Read the model definition and answer for the solid it produces. Units are mm, in the model's axes. A direction names the side the tool comes from. Coordinates: 2 decimals unless noted, no trailing zeros. Order: outer loops, then holes, each group sorted by start corner. A loop starts at its lowest first (then second) coordinate and runs counter-clockwise, first axis right, second up. Notation, with made-up numbers: M 18.5,-26 L 49.5,-26 A13 ccw 49.5,-15 Z; hole C 55.25,2.25 d5. An arc over 180 degrees is marked long. Put each result on its own line as item: value.
Autodesk Inventor part; units mm, degrees
ref_plane "Work Plane1" through (30, 0, 0) normal (0, -0.5, 0.866) x (1, 0, 0)
ref_plane "YZ Plane" through (0, 0, 0) normal (1, 0, 0) x (0, 1, 0)
ref_plane "XZ Plane" through (0, 0, 0) normal (0, 1, 0) x (-1, 0, 0)
sketch "Esquisse1" plane through (0, 0, 0) normal (0, 0, 1) x (1, 0, 0)
  line L0 (-1.1667, 0) -> (20, 0)
  line L1 (20, 0) -> (20, 2.5)
  line L2 (20, 2.5) -> (1.4815, 2.5)
  line L3 (1.4815, 2.5) -> (0.9908, 2.5)
  line L4 (0.9908, 2.5) -> (0, 2.5)
  line L5 (0, 2.5) -> (0, 4.25)
  line L6 (0, 4.25) -> (-5, 4.25)
  line L7 (-5, 4.25) -> (-5, 2.3094)
  line L8 (-5, 2.3094) -> (-2.5, 2.3094)
  line L9 (-2.5, 2.3094) -> (-1.1667, 0)
  line L10 (-10, 0) -> (25, 0)
  line L11 (0, -0.85) -> (0, 5.1)
  line L12 (1.4815, 2.5) -> (0, 2.5) construction
  dimension "d0" = 18.5185
  dimension "d1" = 0.4908
  dimension "d2" = 5
  dimension "d3" = 2.5
  dimension "d4" = 60
  dimension "d5" = 5
  dimension "d6" = 5
  dimension "d7" = 4.6188
  dimension "d8" = 8.5
  dimension "d19" = 20
revolve "Corps" add sketch "Esquisse1" angle 360 about axis through (-1.1667, 0, 0) along (1, 0, 0)
sketch "Esquisse2" plane through (-5, 0, 0) normal (-1, 0, 0) x (0, 0, 1)
  circle A0 centre (0, 0) radius 2.3094
  line L0 (0, -5.95) -> (0, 5.95)
  line L1 (-5.95, 0) -> (5.95, 0)
  line L2 (2.3094, 0) -> (1.1547, -2)
  line L3 (1.1547, -2) -> (-1.1547, -2)
  line L4 (-1.1547, -2) -> (-2.3094, 0)
  line L5 (-2.3094, 0) -> (-1.1547, 2)
  line L6 (-1.1547, 2) -> (1.1547, 2)
  line L7 (1.1547, 2) -> (2.3094, 0)
extrude "Rainure" add sketch "Esquisse2" against normal up to next contours L7 A0 | A0 L2 | L6 L0 A0 | A0 L0 L3 | L0 L6 A0 | A0 L3 L0 | L4 A0 | A0 L5
fillet "Congé2" radius 0.5 1 edges at (-5, -4.25, 0)
thread "Filetage"
chamfer "Chanfrein1" distance 0.4908 distance2 0.4908 1 edges at (20, -2.5, 0) measured on face at (20, -0.7379, -0.3873)
fillet "Congé1" radius 0.2 1 edges at (0, -2.5, 0)
ref_plane "Work Plane1" through (30, 0, 0) normal (0, -0.5, 0.866) x (1, 0, 0)
equation "\"d0\" = GEL"
equation "\"d1\" = GAL"
equation "\"d2\" = KOH"
equation "\"d3\" = INTI"
equation "\"d5\" = GD"
equation "\"d6\" = BDM"
equation "\"d7\" = 1.1547 * SW"
equation "\"d8\" = KOD"
equation "\"d19\" = NLG"
equation "\"d16\" = RR"
equation "\"d12\" = GEL"
equation "\"d14\" = -0.5 * SPD + 0.5 * GD"
equation "\"d15\" = GUL"
equation "\"d29\" = R"
equation "\"GD\" = NND"
equation "\"NLG\" = 20"
equation "\"GEL\" = 18.51848"
equation "\"KOD\" = 8.5"
equation "\"KOH\" = 5"
equation "\"INTI\" = 2.5"
equation "\"GAL\" = 0.61345 * PTC"
equation "\"GUL\" = 0.61345 * PTC"
equation "\"BDM\" = NND"
equation "\"SW\" = 4"
equation "\"RR\" = 0.5"
equation "\"SPD\" = 4.01848"
equation "\"d28\" = R"
equation "\"R\" = 0.2"
equation "\"TOA\" = 30deg"
equation "\"THREADDIA\" = 5"
equation "\"KOD1\" = KOD"
equation "\"PTC\" = 0.8"
equation "\"NND\" = 5"
equation "\"E0\" = 1.155 * SW"
equation "\"GD1\" = THREADDIA - 1.2269 * PTC"
properties part number "ANSI B18.3.1M - M5x0,8 x 20" material "Acier, doux"
Q1. A tool of negligible diameter and unlimited length cuts with its end or side. For faces 1 (the face through (-4, 2, 0)), 2 (the face through (20, 0, 0)), from which of +Z, -Z, +X, -X, +Y, -Y can it reach the whole face along a straight path? Write none if from no direction.
Answers below:
face 1: -X
face 2: +Z, -Z, +X, +Y, -Y
Q2. Consider line 1 along Z through (x, y) = (9.5, 1.5); line 2 along X through (y, z) = (1.75, 3.25); line 3 along Z through (x, y) = (-2, -2.5). Determine where each line is inside the solid, lowest interval first.
Answers below:
line 1: z = -2 to 2
line 2: x = -5 to 0
line 3: z = -3.44 to 3.44
Q3. For a pull along Y with two mould halves and no side action, classify faces 3 (the face through (9.72, -0.54, 2.44)), 4 (the face through (0, 0, -3)), 5 (the face through (-3.68, -0.99, 1.74)) as +Y half, -Y half, draft (parallel to the pull), parting line (faces both ways), or undercut.
Answers below:
face 3: parting line
face 4: draft
face 5: undercut
Q4. Given pin 1 (3 mm diameter, centred on x = 4, y = -2, fed in from +Z); pin 2 (2 mm diameter, centred on y = 3.5, z = 3, fed in from +X); pin 3 (3 mm diameter, centred on x = 10.5, z = 3, fed in from +Y); pin 4 (2 mm diameter, centred on y = -1.5, z = -1.5, fed in from +X), each flat-ended and moving along its own axis, determine where each tip first touches the part or whether it passes through.
Answers below:
pin 1: stops at z = 2.45
pin 2: stops at x = 0
pin 3: stops at y = 2
pin 4: stops at x = 20
Q5. Find section A-A on x = 17.5. Write down the section's boundary in (y, z).
Answers below:
outline: C 0,0 d5
Q6. Find section B-B on x = -1.75. Write down the section's boundary in (y, z).
Answers below:
outline: C 0,0 d8.5; hole C 0,0 d2.02
